```python
from build123d import *
from build123d.topology import SkipClean

# Parameters (mm, degrees)
REVOLVE1_ANGLE     = 180
SKETCH2_R          = 1.5
CUT_EXTRUDE1_DEPTH = 161.623784042
REVOLVE2_ANGLE     = 180
FILLET1_R          = 1


with BuildPart() as part:
    # Sketch1 → Revolve1 (revolve)
    with BuildSketch(Plane.XY):
        with BuildLine():
            Line((-8, 6), (-8, 144))
            ThreePointArc((-8, 144), (-8.94427191, 154.472135955), (0, 160))
            Line((0, 160), (0, -10))
            ThreePointArc((0, -10), (-8.94427191, -4.472135955), (-8, 6))
        make_face()
    revolve(axis=Axis((0, 0, 0), (0, 1, 0)), revolution_arc=REVOLVE1_ANGLE)

    # Sketch2 → Cut-Extrude1 (cut, through all)
    with BuildSketch(Plane(origin=(0, 0, 0), x_dir=(-1, 0, 0), z_dir=(0, 0, -1))):
        Circle(SKETCH2_R)
        with Locations((0, 150)):
            Circle(SKETCH2_R)
    extrude(amount=-CUT_EXTRUDE1_DEPTH, mode=Mode.SUBTRACT)

    # Sketch3 → Revolve2 (revolve)
    with SkipClean():  # the faces are left unmerged after this step: merging them gives an invalid solid
        with BuildSketch(Plane(origin=(0, 0, 0), x_dir=(-1, 0, 0), z_dir=(0, 0, -1))):
            with BuildLine():
                Line((0, 140), (0, 10))
                ThreePointArc((0, 10), (4.472135955, 8.94427191), (8, 6))
                Line((8, 6), (8, 144))
                ThreePointArc((8, 144), (4.472135955, 141.05572809), (0, 140))
            make_face()
        revolve(axis=Axis((0, 150, 0), (0, -1, 0)), revolution_arc=REVOLVE2_ANGLE)

    # Fillet1
    # the kernel refuses this fillet: 1 mm, written as the material it adds along each edge
    with BuildSketch(Plane(origin=(0, 6, 0), x_dir=(-1, 0, 0), z_dir=(0, 0, -1))) as fillet1_piece_1:
        with BuildLine():
            CenterArc((9, 0.32455532), FILLET1_R, 180, 35.096801228)
            Line((8, 0.32455532), (8, 0))
            ThreePointArc((8, 0), (8.091877748, -0.124498786), (8.181818182, -0.250404254))
        make_face()
    revolve(axis=Axis((0, 6, 0), (0, 1, 0)), revolution_arc=180)
    with BuildSketch(Plane(origin=(0, 144, 0), x_dir=(-1, 0, 0), z_dir=(0, 0, -1))) as fillet1_piece_2:
        with BuildLine():
            CenterArc((9, -0.32455532), FILLET1_R, 144.903198772, 35.096801228)
            ThreePointArc((8.181818182, 0.250404254), (8.091877748, 0.124498786), (8, 0))
            Line((8, 0), (8, -0.32455532))
        make_face()
    revolve(axis=Axis((0, 144, 0), (0, 1, 0)), revolution_arc=180)


solid = part.part
```
The model under review builds one solid part; all positions refer to its coordinate system, in mm. Round coordinates to 2 decimals unless told otherwise and drop trailing zeros. Loops run counter-clockwise (first coordinate to the right, second up) from the corner with the lowest first, then second, coordinate; pieces in that order, holes last. Notation, with made-up numbers: (-26, 54) - (-16, 54) arc R8 cw to (-16, 66) - close; hole circle Ø3 at (36.5, 33.5). An arc over 180 degrees is marked (long way). Use a Markdown table: item, result. Add a question column.
Q1. Add section C-C (z = -4.75). State the section outline as (x, y) points.
Q2. Add section A-A (y = 150). State the section outline as (x, z) points.
Q3. Add section B-B (y = 28). State the section outline as (x, z) points, plus the area to 3 significant figures.
Q4. Add section D-D (z = 2.75). State how many separate pieces and enclosed holes the cut face has, plus the area to 3 significant figures.
Q5. For probe 1 along X at (y, z) = (150, 6); probe 2 along Y at (x, z) = (0, 3.5); probe 3 along Y at (x, z) = (0, 3), list the stretches that pass through material, from the lowest coordinate up.
Q6. Insertion check: pin 1 Ø4 at (x, z) = (7, -4) entering from +Y; pin 2 Ø3 at (y, z) = (128.5, 1) entering from -X; pin 3 Ø6 at (x, y) = (2.5, 152.5) entering from -Z. Each pin has a flat end and moves straight along its axis. Give the tip position at first contact, or say it passes through.
Worked answers:
| question | item | result |
|---|---|---|
| 1 | outline | (-6.44, 6) arc R8.8 cw to (6.44, 6) - (6.44, 144) arc R8.8 cw to (-6.44, 144) - close |
| 2 | outline | (-10, 0) - (-1.5, 0) - (-1.5, 9.89) arc R10 ccw to start; (1.5, 0) - (10, 0) arc R10 ccw to (1.5, 9.89) - close |
| 3 | outline | circle Ø16 at (0, 0) |
| 3 | area | 201 mm² |
| 4 | separate pieces | 1 |
| 4 | enclosed holes | 2 |
| 4 | area | 2,560 mm² |
| 5 | probe 1 | -8 to -1.5, 1.5 to 8 |
| 5 | probe 2 | -9.37 to -1.5, 1.5 to 148.5, 151.5 to 159.37 |
| 5 | probe 3 | -9.54 to -1.5, 1.5 to 148.5, 151.5 to 159.54 |
| 6 | pin 1 | y = 144 |
| 6 | pin 2 | x = -8 |
| 6 | pin 3 | z = 0 |
